For this review, take the finished solid that the model builds, in its own axes (mm). Face numbers are marked on the shaded views. A direction names the side the tool comes from. Give positions to 0.01 mm unless a question says otherwise; leave off trailing zeros. Order: outer loops, then holes, each group sorted by start corner. A loop starts at its lowest first (then second) coordinate and runs counter-clockwise, first axis right, second up. Notation, with made-up numbers: (74, -37) -> (109, -37) arc R25 cw to (109, -24) -> close; hole circle Ø8 at (-31, 51.25). An arc over 180 degrees is marked (long way). Use CSV: the item, a comma, the result in double quotes. Start each with the question number.
```python
from build123d import *


with BuildPart() as obj1:
    # Sketch177 → Revolution009 (revolve)
    with BuildSketch(Plane.XY):
        with BuildLine():
            Line((0, 49), (10, 49))
            Line((10, 49), (10, 41))
            Line((10, 41), (9.75, 41))
            Line((9.75, 41), (9.75, 37))
            Line((9.75, 37), (6, 37))
            ThreePointArc((6, 37), (5.292892, 36.707106), (5, 35.999997))
            Line((5, 35.999997), (5, 16))
            ThreePointArc((5, 16), (5.292893, 15.292893), (6, 15))
            Line((6, 15), (8.25, 15))
            Line((8.25, 15), (8.25, 0))
            Line((8.25, 0), (0, 0))
            Line((0, 0), (0, 49))
        make_face()
    revolve(axis=Axis((0, 0, 0), (1, 0, 0)))


with BuildPart() as wheel:
    # Part__Mirroring010: instance of obj1
    add(obj1.part.mirror(Plane(origin=(0, 0, 0), x_dir=(0, -1, 0), z_dir=(1, 0, 0))))

    # Fusion004020026: union obj1
    add(obj1.part)


with BuildPart() as wheel_1:
    # Fusion004020026 placement: moved
    add(wheel.part.moved(Location((65, 0, 0))))


solid = wheel_1.part
```
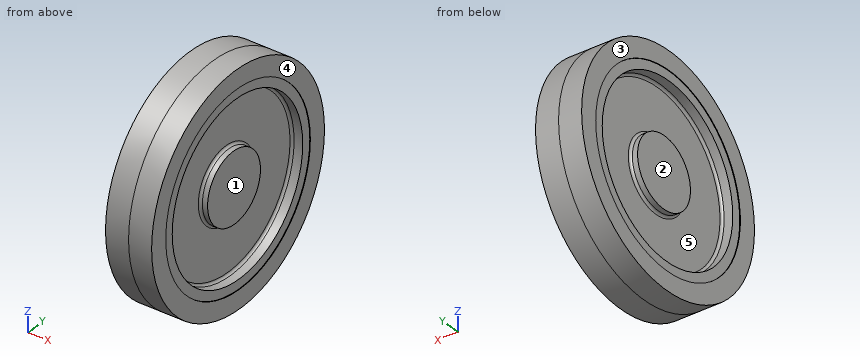
1. For the marked faces 1, 2 and 3, list the 3-axis set-ups (+Z, -Z, +X, -X, +Y, -Y) from which the entire face can be reached by the end or side of a thin tool; tool diameter is ignored.
2. Consider section A-A (x = 67.25). State the section outline as (y, z) points, plus the area to 3 significant figures.
3. Clearance check with flat-ended pins moving along their axes: P1, Ø6, axis at x = 68.5, y = 26.5, coming from the +Z side; P2, Ø4, axis at y = 24.5, z = -6, coming from the +X side; P3, Ø8, axis at x = 62.5, z = -32, coming from the +Y side; P4, Ø10, axis at y = 33, z = -21.5, coming from the +X side. State where each tip first meets the part, or that it passes through.
4. Draft analysis for pull direction Y (two halves, no side actions). For the marked faces 4 and 5, state which applies: +Y half, -Y half, draft (parallel to the pull), parting line (faces both ways), or undercut.
5. To check wall thickness, follow L1, parallel to Z at x = 57.6, y = 0; L2, parallel to Z at x = 72.5, y = 10; L3, parallel to Z at x = 74.8, y = 0. State the ranges of each line that lie inside material, in increasing order. Write a range as [from, to].
Answer list:
1,face 1,"+X"
1,face 2,"-X"
1,face 3,"+Z, -Z, -X, +Y, -Y"
2,outline,"circle Ø98 at (0, 0)"
2,area,"7,540 mm2"
3,P1,"z = 43"
3,P2,"x = 70"
3,P3,"y = 40.21"
3,P4,"x = 75"
4,face 4,"draft"
4,face 5,"undercut"
5,L1,"[-49, -37], [-15, 15], [37, 49]"
5,L2,"[-47.97, -35.62], [-11.18, 11.18], [35.62, 47.97]"
5,L3,"[-49, -41], [41, 49]"
